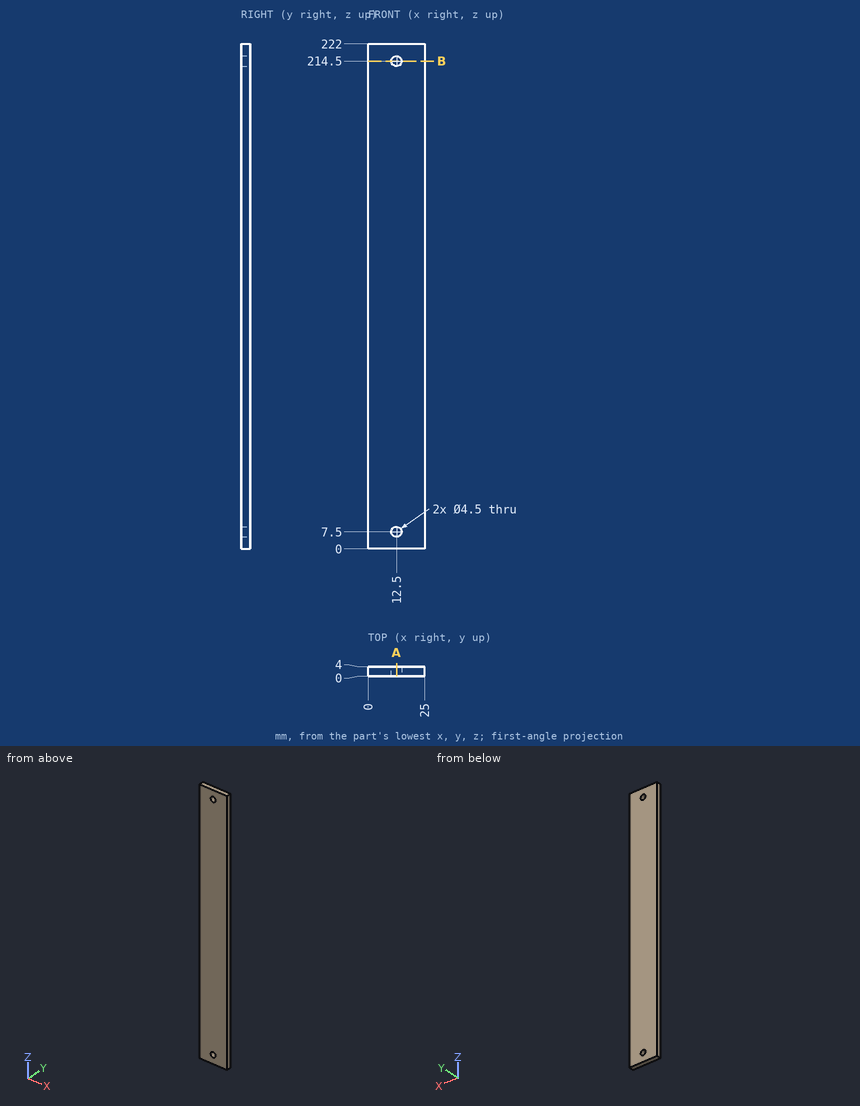
Geometry: see drawing. Coordinates: mm, zero at the bounding-box minimum. Give positions to 0.01 mm unless a question says otherwise; leave off trailing zeros. Order: outer loops, then holes, each group sorted by start corner. A loop starts at its lowest first (then second) coordinate and runs counter-clockwise, first axis right, second up. Notation, with made-up numbers: (49, 8.5) -> (54, 8.5) arc R26 ccw to (54, 40.5) -> close; hole circle Ø5 at (-25.75, 30). An arc over 180 degrees is marked (long way). Write each question's results on one line, items separated by ' | '. Start each with the question number.
1) First-contact query: pin 1 (6 mm diameter, centred on x = 12.5, z = 7.5, fed in from +Y). Flat tip, straight axial feed; report the tip coordinate or a pass-through.
2) Section B-B (z = 214.5). Return loops of the section in (x, y).
3) Section A-A (x = 12.5). Return loops of the section in (y, z).
4) Line query: line 1 (Z direction, x = 12.5, y = 0.95); line 2 (X direction, y = 2.7, z = 214.5). Output: solid intervals per line, ascending. Write a range as from..to.
Calculated:
1) pin 1: y = 4
2) outline: (0, 0) -> (10.25, 0) -> (10.25, 4) -> (0, 4) -> close; (14.75, 0) -> (25, 0) -> (25, 4) -> (14.75, 4) -> close
3) outline: (0, 0) -> (4, 0) -> (4, 5.25) -> (0, 5.25) -> close; (0, 9.75) -> (4, 9.75) -> (4, 212.25) -> (0, 212.25) -> close; (0, 216.75) -> (4, 216.75) -> (4, 222) -> (0, 222) -> close
4) line 1: 0..5.25, 9.75..212.25, 216.75..222 | line 2: 0..10.25, 14.75..25
